Could you check a few things on this drawing? It's one solid part, dimensions in mm from its lowest x, y, z. Coordinates: 2 decimals unless noted, no trailing zeros. Write each loop counter-clockwise with the first axis right and the second up, starting at its lowest first coordinate (ties: lowest second). Pieces come first, ordered by that corner, then holes. Notation, with made-up numbers: (-23.75, 80) - (29.25, 80) arc R16 cw to (29.25, 107) - close; hole circle Ø1 at (-37.5, 56). An arc over 180 degrees is marked (long way). Use one line per item in the form item = value. Start each with the question number.
(1) If we section it at B-B on x = 14.22: Please give me the cut outline in (y, z) (3 decimals), then the cut area to 3 significant figures.
(2) If we section it at A-A on y = 1.05: Please give me the cut outline in (x, z) (3 decimals).
(3) If we section it at D-D on x = 18: Please give me the cut outline in (y, z) (3 decimals), then the cut area to 3 significant figures.
(4) For pin 1 Ø0.6 at (x, y) = (17, 1) entering from -Z; pin 2 Ø0.6 at (y, z) = (1, 17) entering from +X; pin 3 Ø0.6 at (x, y) = (13, 1) entering from +Z, each with a flat end and sliding along its axis, tell me the tip position at first contact or that it passes through.
(5) If we section it at C-C on z = 11.5: Please give me the cut outline in (x, y) (3 decimals), then the cut area to 3 significant figures.
(6) If I drill on probe 1 along Z at (x, y) = (16, 1.2) (3 decimals); probe 2 along Z at (x, y) = (13.75, 0.4) (3 decimals); probe 3 along X at (y, z) = (0.2, 16.5) (3 decimals), over which ranges is the centre line in solid material (lowest first)? Write a range as from..to.
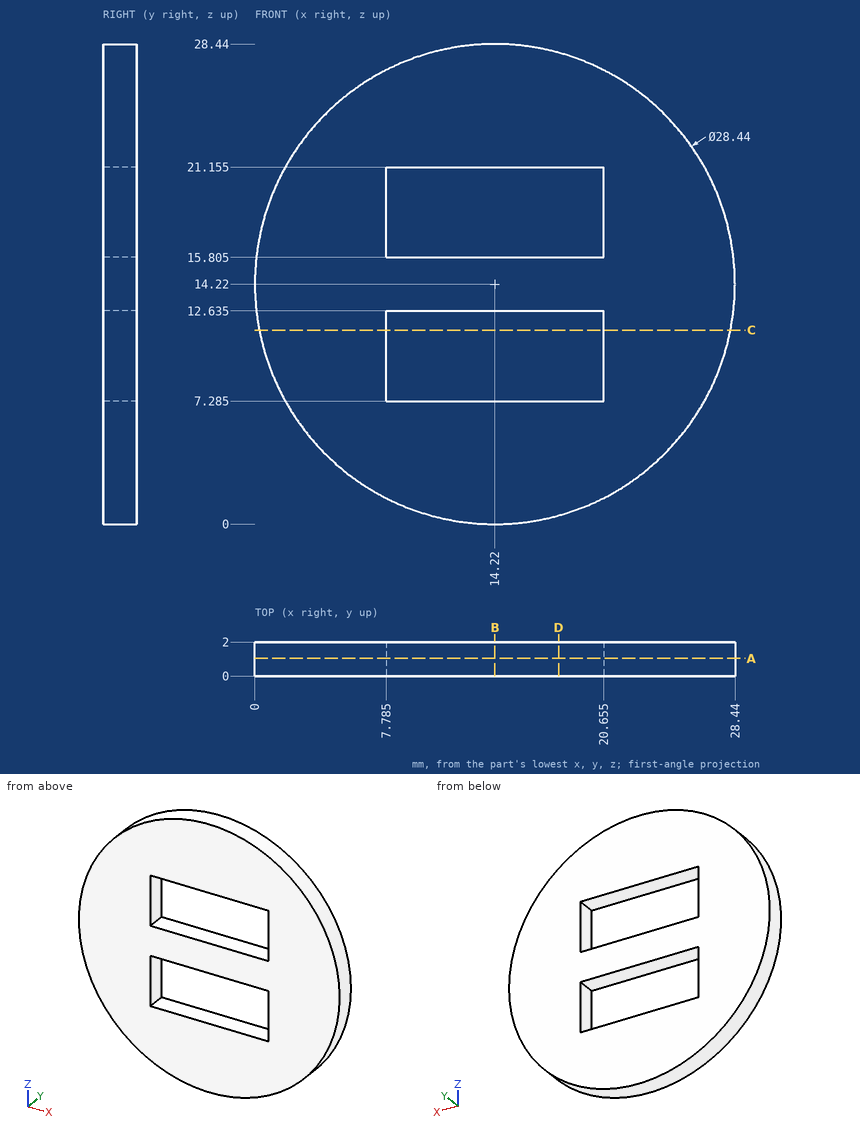
Reported:
q1.outline = (0, 0) - (2, 0) - (2, 7.285) - (0, 7.285) - close; (0, 12.635) - (2, 12.635) - (2, 15.805) - (0, 15.805) - close; (0, 21.155) - (2, 21.155) - (2, 28.44) - (0, 28.44) - close
q1.area = 35.5 mm2
q2.outline = circle Ø28.44 at (14.22, 14.22); hole (7.785, 7.285) - (20.655, 7.285) - (20.655, 12.635) - (7.785, 12.635) - close; hole (7.785, 15.805) - (20.655, 15.805) - (20.655, 21.155) - (7.785, 21.155) - close
q3.outline = (0, 0.512) - (2, 0.512) - (2, 7.285) - (0, 7.285) - close; (0, 12.635) - (2, 12.635) - (2, 15.805) - (0, 15.805) - close; (0, 21.155) - (2, 21.155) - (2, 27.928) - (0, 27.928) - close
q3.area = 33.4 mm2
q4.pin_1 = 0.22
q4.pin_2 = 28.22
q4.pin_3 = 28.41
q5.outline = (0.263, 0) - (7.785, 0) - (7.785, 2) - (0.263, 2) - close; (20.655, 0) - (28.177, 0) - (28.177, 2) - (20.655, 2) - close
q5.area = 30.1 mm2
q6.probe_1 = 0.112..7.285, 12.635..15.805, 21.155..28.328
q6.probe_2 = 0.008..7.285, 12.635..15.805, 21.155..28.432
q6.probe_3 = 0.184..7.785, 20.655..28.256
